Geometry check sheet. Reference: the model listing, model coordinates, mm. A direction names the side the tool comes from. Give positions to 0.01 mm unless a question says otherwise; leave off trailing zeros. Loops run counter-clockwise (first coordinate to the right, second up) from the corner with the lowest first, then second, coordinate; pieces in that order, holes last.
1. Cross-section at D-D, the plane z = -1.75. Record the cut outline in (x, y), plus the area to 3 significant figures.
2. Cross-section at A-A, the plane z = -5.25. Record the cut outline in (x, y).
3. Tool access check on faces 1 (the flat face through (-6.19, 0.66, 0.28)), 2 (the flat face through (0, -2, 4.5)), 3 (the cylindrical face through (-1.9, 0.5, 3.8)), 4 (the cylindrical face through (-1.9, 0.9, 3.8)), 5 (the flat face through (0, -2, 4.2)). Record the directions out of +Z, -Z, +X, -X, +Y, -Y that give a thin tool (end or side, any length) a straight path to the whole face; none if there is none.
4. Cross-section at C-C, the plane y = -2.2. Record the cut outline in (x, z).
5. Release check for a two-part mould opening along Z. For faces 6 (the flat face through (0, 0.4, 1.9)), 7 (the flat face through (-6.19, 0.94, 0.32)), 8 (the flat face through (6.19, 0.66, 0.28)) record: +Z half, -Z half, draft (parallel to the pull), parting line (faces both ways), or undercut.
6. Cross-section at B-B, the plane x = -6.25. Record the cut outline in (y, z), plus the area to 3 significant figures.
7. Material ranges on L1, parallel to Y at x = 0.5, z = 3.25; L2, parallel to Y at x = 3.25, z = 5; L3, parallel to X at y = -2.85, z = 3.5, recorded low to high.
8. Go/stop test with flat-tipped pins: pin 1 Ø0.5 at (y, z) = (1, 0.5) entering from -X; pin 2 Ø1.5 at (x, z) = (-2.5, -0.5) entering from -Y; pin 3 Ø3 at (y, z) = (-1, 4) entering from +X. Record where each tip stops, or that it passes through.
from build123d import *

# Parameters (mm, degrees)
SKETCH1_W               = 15
SKETCH1_H               = 13
BASE_DEPTH              = 0.3
SKETCH7_W               = 1.8
SKETCH7_H               = 2.4
LOCKING_CLAMP_CUT_DEPTH = 10.92924972
LOCKING_CLAMP_DEPTH     = 0.8
SPRING_CLASP_DEPTH      = 0.2
WIRE_CONNECTION_DEPTH   = 1
SKETCH14_W              = 9
SKETCH14_H              = 2
BOTTOM_SLOT_CUT_DEPTH   = 11.816191566
TS_F_R                  = 1
BS_F_R                  = 4
WC_F_R                  = 0.5
BSC_F_R                 = 0.4


with BuildPart() as part:
    # Sketch1 → BASE (new body)
    with BuildSketch(Plane(origin=(0, 0, 0), x_dir=(1, 0, 0), z_dir=(0, 1, 0))):
        Rectangle(SKETCH1_W, SKETCH1_H)
    extrude(amount=BASE_DEPTH)

    # Sketch7 → LOCKING CLAMP CUT (cut, through all)
    with BuildSketch(Plane(origin=(0, 0.3, 0), x_dir=(1, 0, 0), z_dir=(0, 1, 0))):
        with Locations((6.2, -0.3)):
            Rectangle(SKETCH7_W, SKETCH7_H)
    locking_clamp_cut = extrude(amount=-LOCKING_CLAMP_CUT_DEPTH, mode=Mode.SUBTRACT)

    # Sketch9 → LOCKING CLAMP (add, symmetric)
    with BuildSketch(Plane.ZY.offset(-6.2)):
        Polygon((1.5, 0.3), (-0.9, 1.6), (-0.9, 1.3), (1.5, 0), align=None)
    locking_clamp = extrude(amount=LOCKING_CLAMP_DEPTH, both=True)

    # LC M: LOCKING CLAMP CUT, LOCKING CLAMP across plane
    add(locking_clamp_cut.mirror(Plane(origin=(0, 0, 0), x_dir=(0, 0, 1), z_dir=(1, 0, 0))), mode=Mode.SUBTRACT)
    add(locking_clamp.mirror(Plane(origin=(0, 0, 0), x_dir=(0, 0, 1), z_dir=(1, 0, 0))))

    # Sketch11 → SPRING CLASP (add, symmetric)
    with BuildSketch(Plane(origin=(0.95, 0, 0.95), x_dir=(-0.7071067811865436, 0, 0.7071067811865516), z_dir=(-0.7071067811865516, 0, -0.7071067811865436))):
        with BuildLine():
            Line((5.343502884, 0), (4.635110863, 0))
            ThreePointArc((4.635110863, 0), (4.57056114, 0.023623738), (4.536509533, 0.083333333))
            ThreePointArc((4.536509533, 0.083333333), (4.043502884, 0.5), (3.550496236, 0.083333333))
            ThreePointArc((3.550496236, 0.083333333), (3.516444628, 0.023623738), (3.451894906, 0))
            Line((3.451894906, 0), (-0.764889137, 0))
            ThreePointArc((-0.764889137, 0), (-0.82943886, 0.023623738), (-0.863490467, 0.083333333))
            ThreePointArc((-0.863490467, 0.083333333), (-1.356497116, 0.5), (-1.849503764, 0.083333333))
            ThreePointArc((-1.849503764, 0.083333333), (-1.883555372, 0.023623738), (-1.948105094, 0))
            Line((-1.948105094, 0), (-2.656497116, 0))
            Line((-2.656497116, 0), (-2.656497116, 0.4))
            Line((-2.656497116, 0.4), (-2.162722891, 0.4))
            ThreePointArc((-2.162722891, 0.4), (-1.356497116, 0.9), (-0.550271341, 0.4))
            Line((-0.550271341, 0.4), (3.237277109, 0.4))
            ThreePointArc((3.237277109, 0.4), (4.043502884, 0.9), (4.849728659, 0.4))
            Line((4.849728659, 0.4), (5.343502884, 0.4))
            Line((5.343502884, 0.4), (5.343502884, 0))
        make_face()
    extrude(amount=SPRING_CLASP_DEPTH, both=True)

    # Sketch13 → WIRE CONNECTION (add, symmetric)
    with BuildSketch(Plane(origin=(0, 0, 0), x_dir=(0, 0, -1), z_dir=(1, 0, 0))):
        Polygon((-6.5, 0), (-2.5, -4), (-2.2, -4), (-6.2, 0), align=None)
    extrude(amount=WIRE_CONNECTION_DEPTH, both=True)

    # Sketch14 → BOTTOM SLOT CUT (cut, through all)
    with BuildSketch(Plane(origin=(0, 0.3, 0), x_dir=(1, 0, 0), z_dir=(0, 1, 0))):
        with Locations((0, 5.5)):
            Rectangle(SKETCH14_W, SKETCH14_H)
    extrude(amount=-BOTTOM_SLOT_CUT_DEPTH, mode=Mode.SUBTRACT)

    # TS F
    ts_f_edges = [part.edges().sort_by_distance(p)[0] for p in [
        (-7.5, 0.15, -6.5),
        (7.5, 0.15, -6.5),
    ]]
    fillet(ts_f_edges, radius=TS_F_R)

    # BS F
    bs_f_edges = [part.edges().sort_by_distance(p)[0] for p in [
        (7.5, 0.15, 6.5),
        (-7.5, 0.15, 6.5),
    ]]
    fillet(bs_f_edges, radius=BS_F_R)

    # WC F
    # the kernel refuses this fillet: 0.5 mm, written as the material it takes off along each edge
    with BuildSketch(Plane(origin=(-1, -4, 3.75), x_dir=(0, 1, 0), z_dir=(0, 0, -1))) as wc_f_piece_1:
        with BuildLine():
            CenterArc((WC_F_R, WC_F_R), WC_F_R, 180, 90)
            Line((0, WC_F_R), (0, 0))
            Line((0, 0), (WC_F_R, 0))
        make_face()
    extrude(amount=2.8, mode=Mode.SUBTRACT)
    with BuildSketch(Plane(origin=(1, -4, 3.75), x_dir=(0, 1, 0), z_dir=(0, 0, -1))) as wc_f_piece_2:
        with BuildLine():
            CenterArc((WC_F_R, -WC_F_R), WC_F_R, 90, 90)
            Line((0, -WC_F_R), (0, 0))
            Line((0, 0), (WC_F_R, 0))
        make_face()
    extrude(amount=2.8, mode=Mode.SUBTRACT)

    # BSC F
    bsc_f_edges = [part.edges().sort_by_distance(p)[0] for p in [
        (4.5, 0.15, -6.5),
        (-4.5, 0.15, -6.5),
        (4.5, 0.15, -4.5),
        (-4.5, 0.15, -4.5),
    ]]
    fillet(bsc_f_edges, radius=BSC_F_R)


solid = part.part
Result:
1. outline: (-7.5, 0) - (7.5, 0) - (7.5, 0.3) - (-7.5, 0.3) - close
1. area: 4.50 mm2
2. outline: (-7.5, 0) - (-4.5, 0) - (-4.5, 0.3) - (-7.5, 0.3) - close; (4.5, 0) - (7.5, 0) - (7.5, 0.3) - (4.5, 0.3) - close
3. face 1: -Y
3. face 2: +Z, +X, -X, -Y
3. face 3: none
3. face 4: +Y
3. face 5: -Z, +X, -X
4. outline: (-1, 4) - (1, 4) - (1, 4.3) - (-1, 4.3) - close
5. face 6: draft
5. face 7: +Z half
5. face 8: undercut
6. outline: (0, -6.5) - (0.3, -6.5) - (0.3, -0.9) - (0, -0.9) - close; (0, 1.5) - (1.3, -0.9) - (1.6, -0.9) - (0.3, 1.5) - (0.3, 5.4) - (0, 5.4) - close
6. area: 3.57 mm2
7. L1: y = -3.25 to -2.95, 0 to 0.3
7. L2: y = 0 to 0.3
7. L3: x = -1 to 1
8. pin 1: stops at x = -7
8. pin 2: stops at y = 0
8. pin 3: stops at x = 7.48
